from build123d import *

# Parameters (mm, degrees)
BASE_FLANGE1_DEPTH = 2
SKETCH8_R          = 2
CUT_EXTRUDE1_DEPTH = 2


# Sheet-metal steps are written as plain solids
with BuildPart() as part:
    # Sketch3 → Base-Flange1 (new body)
    with BuildSketch(Plane(origin=(0, 0, 0), x_dir=(1, 0, 0), z_dir=(0, 1, 0))):
        with BuildLine():
            Line((-29.187643745, 8.908278482), (-29.187643745, 25.875))
            Line((-29.187643745, 25.875), (-29.187643745, 50.875))
            Line((-29.187643745, 50.875), (-19.187643745, 50.875))
            Line((-19.187643745, 50.875), (-19.187643745, 25.875))
            Line((-19.187643745, 25.875), (29.187643745, 25.875))
            Line((29.187643745, 25.875), (29.187643745, 8.908278482))
            ThreePointArc((29.187643745, 8.908278482), (22.95, 10.875), (16.712356255, 8.908278482))
            ThreePointArc((16.712356255, 8.908278482), (11.475, 6.552640597), (6.237643745, 8.908278482))
            ThreePointArc((6.237643745, 8.908278482), (0, 10.875), (-6.237643745, 8.908278482))
            ThreePointArc((-6.237643745, 8.908278482), (-11.475, 6.552640597), (-16.712356255, 8.908278482))
            ThreePointArc((-16.712356255, 8.908278482), (-22.95, 10.875), (-29.187643745, 8.908278482))
        make_face()
    extrude(amount=-BASE_FLANGE1_DEPTH)

    # Sketch8 → Cut-Extrude1 (cut)
    with BuildSketch(Plane(origin=(0, 0, 0), x_dir=(1, 0, 0), z_dir=(0, 1, 0))):
        with Locations(Location((-24.187643745, 44.375, 0), (0, 0, 270))):
            Circle(SKETCH8_R)
        with Locations(Location((-24.187643745, 34.875, 0), (0, 0, 270))):
            Circle(SKETCH8_R)
    extrude(amount=-CUT_EXTRUDE1_DEPTH, mode=Mode.SUBTRACT)


solid = part.part
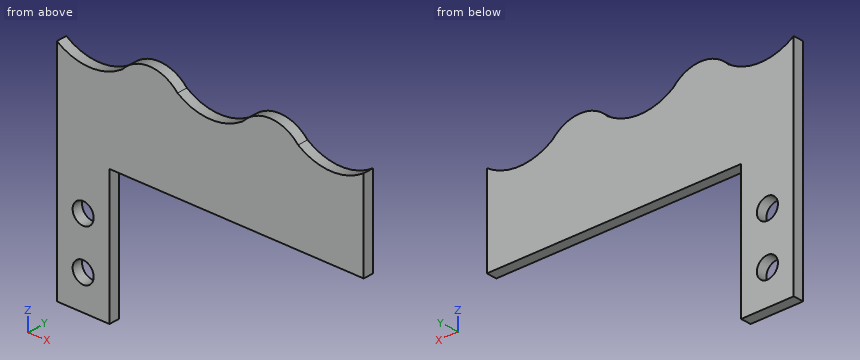
Work out the finished part from the listing and answer in its coordinate system (mm). Coordinates: 2 decimals unless noted, no trailing zeros. Order: outer loops, then holes, each group sorted by start corner. A loop starts at its lowest first (then second) coordinate and runs counter-clockwise, first axis right, second up. Notation, with made-up numbers: (34, 15.25) - (86, 15.25) arc R23 cw to (86, 54.25) - close; hole circle Ø8 at (-25, 73.25). An arc over 180 degrees is marked (long way). Put each result on its own line as item: value. Start each with the question number.
1) Find the intervals of material crossed by line 1 (Z direction, x = -23.5, y = -1.05) (3 decimals); line 2 (Z direction, x = -26, y = -0.7) (3 decimals); line 3 (X direction, y = -0.85, z = -28), in increasing order. Write a range as from..to.
2) Find section D-D (z = -29). Give the vertices of the cut face in (x, y), plus the area to 3 significant figures.
3) Find section C-C (x = 14.5). Give the vertices of the cut face in (y, z) (3 decimals).
4) Find section B-B (y = -0.3). Give the vertices of the cut face in (x, z) (3 decimals).
5) Flat-ended cylindrical pins translate along their axes: pin 1 (3.5 mm diameter, centred on x = -24.19, z = -44.38, fed in from +Y); pin 2 (0.6 mm diameter, centred on y = -1.5, z = -36, fed in from +X). Find the tip coordinate at first contact, or state that the pin passes through.
6) Find section A-A (x = -23.5). Give the vertices of the cut face in (y, z) (3 decimals).
Results list:
1. line 1: z = -50.875..-46.253, -42.497..-36.753, -32.997..-10.861
1. line 2: z = -50.875..-45.221, -43.529..-35.721, -34.029..-10.439
1. line 3: x = -29.19..-19.19
2. outline: (-29.19, -2) - (-19.19, -2) - (-19.19, 0) - (-29.19, 0) - close
2. area: 20.0 mm^2
3. outline: (-2, -25.875) - (0, -25.875) - (0, -7.24) - (-2, -7.24) - close
4. outline: (-29.188, -50.875) - (-19.188, -50.875) - (-19.188, -25.875) - (29.188, -25.875) - (29.188, -8.908) arc R10.875 cw to (16.712, -8.908) arc R7 ccw to (6.238, -8.908) arc R10.875 cw to (-6.238, -8.908) arc R7 ccw to (-16.712, -8.908) arc R10.875 cw to (-29.188, -8.908) - close; hole circle Ø4 at (-24.188, -44.375); hole circle Ø4 at (-24.188, -34.875)
5. pin 1: passes through
5. pin 2: stops at x = -19.19
6. outline: (-2, -50.875) - (0, -50.875) - (0, -46.253) - (-2, -46.253) - close; (-2, -42.497) - (0, -42.497) - (0, -36.753) - (-2, -36.753) - close; (-2, -32.997) - (0, -32.997) - (0, -10.861) - (-2, -10.861) - close
